Can you work these out from the drawing? Everything is in mm from the part's minimum corner. A direction names the side the tool comes from. Round coordinates to 2 decimals unless told otherwise and drop trailing zeros. Order: outer loops, then holes, each group sorted by start corner. A loop starts at its lowest first (then second) coordinate and runs counter-clockwise, first axis right, second up. Notation, with made-up numbers: (-5, 77) -> (18, 77) arc R18 cw to (18, 86) -> close; hole circle Ø4 at (7, 79.25). An arc over 180 degrees is marked (long way). One line per item, written item: value.
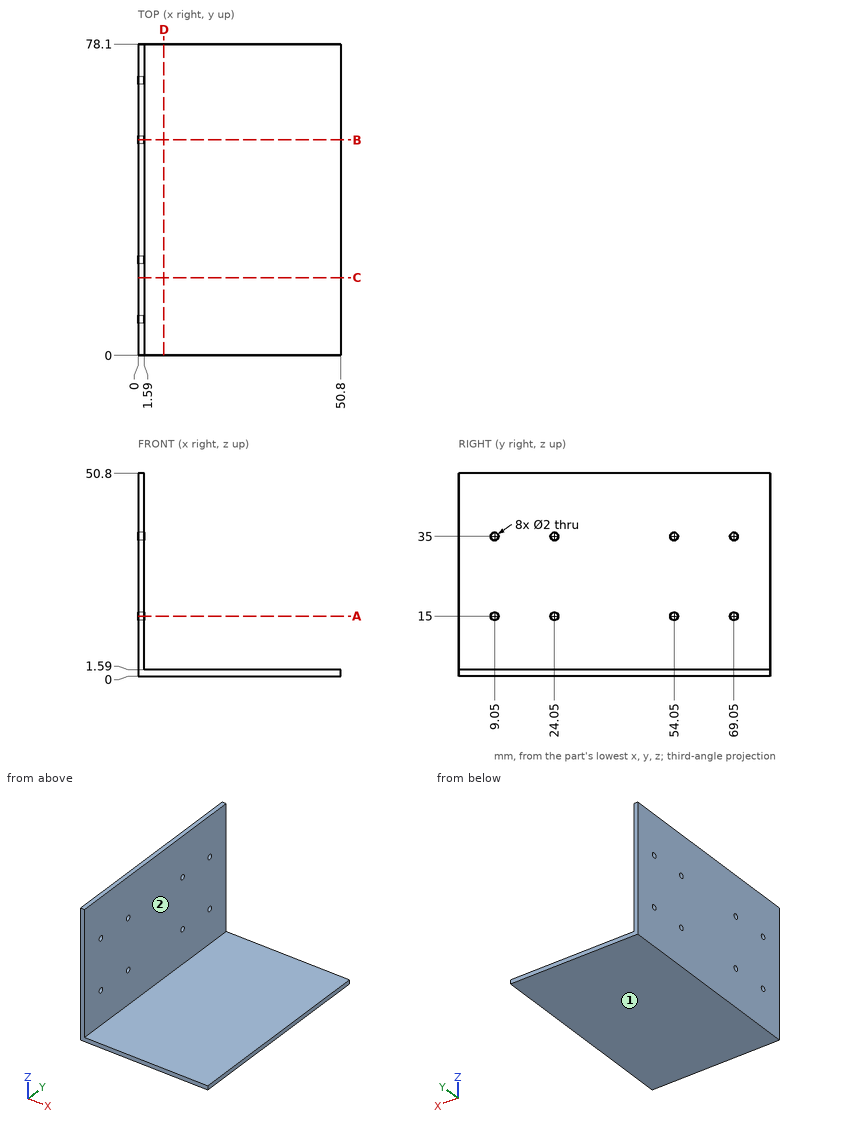
Q1. Please list where these lines run through material, in increasing order: line 1 along Z through (x, y) = (1.1, 69.05); line 2 along Y through (x, z) = (1.1, 35); line 3 along Z through (x, y) = (10, 43).
Answers below:
line 1: 0 to 14, 16 to 34, 36 to 50.8
line 2: 0 to 8.05, 10.05 to 23.05, 25.05 to 53.05, 55.05 to 68.05, 70.05 to 78.1
line 3: 0 to 1.59
Q2. I want a section at A-A on z = 15. List the corners of the cut face in (x, y) for me.
Answers below:
outline: (0, 0) -> (1.59, 0) -> (1.59, 8.05) -> (0, 8.05) -> close; (0, 10.05) -> (1.59, 10.05) -> (1.59, 23.05) -> (0, 23.05) -> close; (0, 25.05) -> (1.59, 25.05) -> (1.59, 53.05) -> (0, 53.05) -> close; (0, 55.05) -> (1.59, 55.05) -> (1.59, 68.05) -> (0, 68.05) -> close; (0, 70.05) -> (1.59, 70.05) -> (1.59, 78.1) -> (0, 78.1) -> close
Q3. I want a section at C-C on y = 19.5. List the corners of the cut face in (x, z) for me.
Answers below:
outline: (0, 0) -> (50.8, 0) -> (50.8, 1.59) -> (1.59, 1.59) -> (1.59, 50.8) -> (0, 50.8) -> close
Q4. I want a section at B-B on y = 54.05. List the corners of the cut face in (x, z) for me.
Answers below:
outline: (0, 0) -> (50.8, 0) -> (50.8, 1.59) -> (1.59, 1.59) -> (1.59, 14) -> (0, 14) -> close; (0, 16) -> (1.59, 16) -> (1.59, 34) -> (0, 34) -> close; (0, 36) -> (1.59, 36) -> (1.59, 50.8) -> (0, 50.8) -> close
Q5. Will these pins go through, and if not, where does the flat tip stop? pin 1 Ø2.5 at (y, z) = (54.05, 15) entering from -X; pin 2 Ø1.8 at (y, z) = (9.05, 15) entering from +X; pin 3 Ø15 at (y, z) = (52, 37.5) entering from +X; pin 4 Ø3 at (x, y) = (41, 33) entering from +Z.
Answers below:
pin 1: x = 0
pin 2: through
pin 3: x = 1.59
pin 4: z = 1.59
Q6. On a 3-axis mill with a long thin cutter (end or side, diameter ignored), from which of +Z, -Z, +X, -X, +Y, -Y can I reach the whole of each face in a straight line? I mean the marked faces 1 and 2. Say none if no direction works.
Answers below:
face 1: -Z, +X, -X, +Y, -Y
face 2: +Z, +X, +Y, -Y
Q7. I want a section at D-D on x = 6.5. List the corners of the cut face in (y, z) for me.
Answers below:
outline: (0, 0) -> (78.1, 0) -> (78.1, 1.59) -> (0, 1.59) -> close
